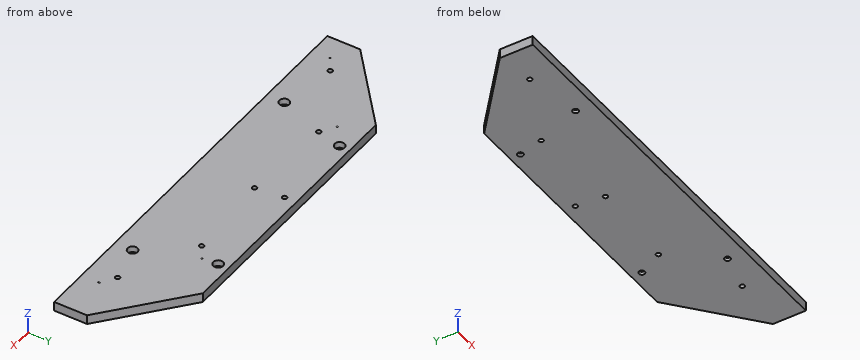
Solid Edge part; units mm, degrees
sketch "Sketch1" plane through (0, 0, 0) normal (0, 0, 1) x (1, 0, 0)
  line L0 (-225, -52.5) -> (225, -52.5)
  line L1 (225, -52.5) -> (225, -17.5)
  line L2 (225, -17.5) -> (142.5, 52.5)
  line L3 (142.5, 52.5) -> (-142.5, 52.5)
  line L4 (-225, -17.5) -> (-142.5, 52.5)
  line L5 (-225, -52.5) -> (-225, -17.5)
  dimension "D1" = 142.5
  dimension "D2" = 225
  dimension "D3" = 225
  dimension "D4" = 225
extrude "Protrusion1" add sketch "Sketch1" along normal blind 10
hole "Hole1" at (-8.4234, 10, 10) direction (0, 0, -1) diameter 4.917 end up to next
hole "Hole2" at (-11.5766, 40, 10) direction (0, 0, -1) diameter 4.917 end up to next
hole "Hole3" at (-185, -23.6057, 10) direction (0, 0, -1) diameter 4.917 end up to next
hole "Hole4" at (-106.5, 15, 10) direction (0, 0, -1) diameter 4.917 end up to next
hole "Hole5" at (86.5, 15, 10) direction (0, 0, -1) diameter 4.917 end up to next
hole "Hole6" at (165, -23.6057, 10) direction (0, 0, -1) diameter 4.917 end up to next
sketch "Sketch2" plane through (0, 0, 10) normal (0, 0, 1) x (1, 0, 0)
  circle A0 centre (-200, -33.6057) radius 1
  circle A1 centre (-121.5, 25) radius 1
  circle A2 centre (101.5, 25) radius 1
  circle A3 centre (180, -33.6057) radius 1
extrude "Mirrormarks" cut sketch "Sketch2" against normal blind 0.1
sketch "Sketch3" plane through (0, 0, 10) normal (0, 0, 1) x (1, 0, 0)
  circle A0 centre (125, -33.6057) radius 5.25
  circle A1 centre (100, 41.3943) radius 5.25
  circle A2 centre (-100, 41.3943) radius 5.25
  circle A3 centre (-125, -33.6057) radius 5.25
extrude "Mounting_screws" cut sketch "Sketch3" against normal blind 6.5
sketch "Sketch4" plane through (-125, 41.3943, 3.5) normal (0, 0, 1) x (1, 0, 0)
  circle A0 centre (25, 0) radius 3.15
  circle A1 centre (225, 0) radius 3.15
  circle A2 centre (250, -75) radius 3.15
  circle A3 centre (0, -75) radius 3.15
extrude "Cutout1" cut sketch "Sketch4" against normal up to next
Here's how the part is built. I have some questions about the finished solid (model axes, mm). Give positions to 0.01 mm unless a question says otherwise; leave off trailing zeros. Loops run counter-clockwise (first coordinate to the right, second up) from the corner with the lowest first, then second, coordinate; pieces in that order, holes last. Notation, with made-up numbers: M 50.5,45 L 89.5,45 A17 cw 89.5,58 Z; hole C -2.75,-37.5 d4. An arc over 180 degrees is marked long. Return JSON: item names as keys, results as strings.
Item 1: Imagine slicing it at B-B on x = -171. List the corners of the cut face in (y, z) for me.
A:
{"outline": "M -52.5,0 L 28.32,0 L 28.32,10 L -52.5,10 Z"}
Item 2: Please list where these lines run through material, in increasing order: line 1 (Y direction, x = -125, z = 1.35); line 2 (X direction, y = 15, z = 6.25); line 3 (X direction, y = -36, z = 4.25).
A:
{"line 1": "y = -52.5 to -36.76, -30.46 to 52.5", "line 2": "x = -186.7 to -108.96, -104.04 to 84.04, 88.96 to 186.7", "line 3": "x = -225 to -129.67, -120.33 to 120.33, 129.67 to 225"}
Item 3: I'm going to push flat-ended pins straight in: pin 1 Ø3 at (x, y) = (-123, -32.5) entering from +Z; pin 2 Ø3 at (x, y) = (86.5, 15) entering from +Z; pin 3 Ø1.6 at (x, y) = (-121.5, 25) entering from +Z. Where does each tip first touch, or does it pass through?
A:
{"pin 1": "stops at z = 3.5", "pin 2": "passes through", "pin 3": "stops at z = 9.9"}
Item 4: Imagine slicing it at A-A on z = 8. State how many separate pieces and enclosed holes the cut face has, then the cut area to 3 significant figures.
A:
{"separate pieces": "1", "enclosed holes": "10", "area": "41,000 mm^2"}
